Part model, mm, in its own coordinate system. Face numbers are marked on the shaded views. A direction names the side the tool comes from. Coordinates: 2 decimals unless noted, no trailing zeros. Loops run counter-clockwise (first coordinate to the right, second up) from the corner with the lowest first, then second, coordinate; pieces in that order, holes last. Notation, with made-up numbers: M 85.5,-35.5 L 89.5,-35.5 A17 ccw 89.5,-20.5 Z; hole C 45.25,-8.75 d9. An arc over 180 degrees is marked long. Use CSV: the item, a comma, the result in double quotes. Start each with the question number.
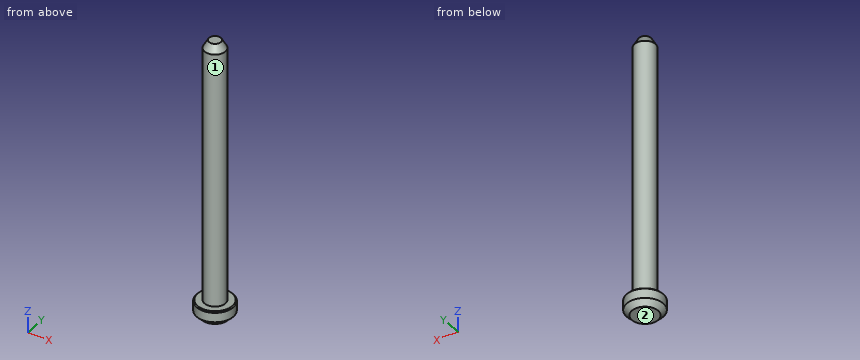
from build123d import *

# Parameters (mm, degrees)
CHAMFER1_SIZE = 0.2


with BuildPart() as part:
    # Sketch1 → Revolve1 (revolve)
    with BuildSketch(Plane(origin=(0, 0, 0), x_dir=(1, 0, 0), z_dir=(0, 1, 0))):
        Polygon((0, 0), (0, 53), (2.5, 53), (3.5, 52), (3.5, 50), (2, 50), (2, 1.5), (1.133974596, 0), align=None)
    revolve(axis=Axis((0, 0, 0), (0, 0, 1)))

    # Chamfer1
    chamfer1_edges = [part.edges().sort_by_distance(p)[0] for p in [
        (-3.5, 0, -50),
    ]]
    chamfer(chamfer1_edges, length=CHAMFER1_SIZE)


solid = part.part
1. Slice it at A-A, the plane y = 0. List the corners of the cut face in (x, z), and give its area (3 significant figures).
2. Tool access for the marked faces 1 and 2: list every direction of +Z, -Z, +X, -X, +Y, -Y with a clear straight run to the whole face (end or side of a thin tool).
3. Wall check: probe 1 along Z at (x, y) = (1.5, 1.75); probe 2 along X at (y, z) = (-0.5, -26); probe 3 along Z at (x, y) = (-1, 2.75). Give the ranges that are in metal, low to high.
4. Pin check, flat tips, straight feed: pin 1 (1 mm diameter, centred on x = 1.5, z = -46, fed in from -Y); pin 2 (1 mm diameter, centred on y = -1, z = -20, fed in from -X); pin 3 (3 mm diameter, centred on x = 1.5, z = -28, fed in from +Y). Stop position of each tip, or through.
5. Slice it at C-C, the plane z = -22. List the corners of the cut face in (x, y), and give its area (3 significant figures).
Found:
1,outline,"M -3.5,-52 L -2.5,-53 L 2.5,-53 L 3.5,-52 L 3.5,-50.2 L 3.3,-50 L 2,-50 L 2,-1.5 L 1.13,0 L -1.13,0 L -2,-1.5 L -2,-50 L -3.3,-50 L -3.5,-50.2 Z"
1,area,"219 mm^2"
2,face 1,"+Z"
2,face 2,"-Z, +X, -X, +Y, -Y"
3,probe 1,"-53 to -50"
3,probe 2,"-1.94 to 1.94"
3,probe 3,"-52.57 to -50"
4,pin 1,"y = -1.73"
4,pin 2,"x = -1.94"
4,pin 3,"y = 2"
5,outline,"C 0,0 d4"
5,area,"12.6 mm^2"
